Verification items for the finished model (mm, model axes). A direction names the side the tool comes from. Give positions to 0.01 mm unless a question says otherwise; leave off trailing zeros. Write each loop counter-clockwise with the first axis right and the second up, starting at its lowest first coordinate (ties: lowest second). Pieces come first, ordered by that corner, then holes. Notation, with made-up numbers: M -18,53 L -10,53 A23 ccw -10,92 Z; hole C 66.5,-38.5 d9. An arc over 180 degrees is marked long. Write item = value, one per line.
Autodesk Fusion 360 part; units mm, degrees
sketch "Sketch1" plane through (0, 0, 0) normal (1, 0, 0) x (0, 0, -1)
  line L0 (0, 0) -> (0, 45)
  line L1 (0, 0) -> (0, -45)
  line L2 (0, 45) -> (37.5, 45)
  line L3 (0, 45) -> (-37.5, 45)
  line L4 (0, -45) -> (37.5, -45)
  line L5 (0, -45) -> (-37.5, -45)
  arc A0 (-37.5, 45) -> (-37.5, -45) centre (79.119, 0) ccw
  arc A1 (37.5, -45) -> (37.5, 45) centre (-79.119, 0) ccw
  dimension "d1" = 45
  dimension "d2" = 45
  dimension "d3" = 37.5
  dimension "d4" = 37.5
  dimension "d5" = 37.5
  dimension "d6" = 37.5
  dimension "d8" = 125
extrude "Extrude1" add sketch "Sketch1" along normal blind 100
extrude "Extrude2" add 1 faces at (100, -15.2642, -14.2806) along direction (1, 0, 0) blind 35 draft -15
sketch "Sketch2" plane through (135, 0, 0) normal (1, 0, 0) x (0, 0, -1)
  line L0 (-30.8786, -35.6218) -> (30.8786, -35.6218)
  arc A0 (30.8786, -35.6218) -> (30.8786, 35.6218) centre (-79.119, 0) ccw
  line L1 (30.8786, 35.6218) -> (-30.8786, 35.6218)
  arc A1 (-30.8786, 35.6218) -> (-30.8786, -35.6218) centre (79.119, 0) ccw
  circle A2 centre (0, 0) radius 34.5
  dimension "d13" = 69
extrude "Extrude3" add sketch "Sketch2" along normal blind 10 contours A2
sketch "Sketch3" plane through (145, 0, 0) normal (1, 0, 0) x (0, 0, -1)
  circle A0 centre (0, 0) radius 34.5
  circle A1 centre (0, 0) radius 31
  dimension "d16" = 62
extrude "Extrude4" add sketch "Sketch3" along normal blind 30 contours A1
sketch "Sketch4" plane through (175, 0, 0) normal (1, 0, 0) x (0, 0, -1)
  circle A0 centre (0, 0) radius 31
  line L0 (0, 0) -> (27, 0)
  circle A1 centre (27, 0) radius 2.5
  circle A2 centre (27, 0) radius 1.5
  dimension "d19" = 27
  dimension "d20" = 5
  dimension "d21" = -1
extrude "Extrude5" add sketch "Sketch4" along normal blind 1 contours A1
pattern_circular "C-Pattern1" count 12 over 360 about axis through (175, 0, 0) along (1, 0, 0) of "Extrude5"
sketch "Sketch5" plane through (175, 0, 0) normal (1, 0, 0) x (0, 0, -1)
  circle A0 centre (27, 0) radius 2.5
  circle A1 centre (0, 0) radius 31
  circle A2 centre (23.3827, 13.5) radius 2.5
  circle A3 centre (13.5, 23.3827) radius 2.5
  circle A4 centre (0, 27) radius 2.5
  circle A5 centre (-13.5, 23.3827) radius 2.5
  circle A6 centre (-23.3827, 13.5) radius 2.5
  circle A7 centre (-27, 0) radius 2.5
  circle A8 centre (-23.3827, -13.5) radius 2.5
  circle A9 centre (-13.5, -23.3827) radius 2.5
  circle A10 centre (0, -27) radius 2.5
  circle A11 centre (13.5, -23.3827) radius 2.5
  circle A12 centre (23.3827, -13.5) radius 2.5
  line L0 (0, 0) -> (16, 0)
  line L1 (16, 0) -> (16, 17)
  line L2 (16, 0) -> (16, -17)
  line L3 (0, 0) -> (0, -8.0593)
  line L4 (-16, 0) -> (-16, 17)
  line L5 (-16, 0) -> (-16, -17)
  arc A13 (16, 17) -> (-16, 17) centre (0, 1.9003) ccw
  arc A14 (-16, -17) -> (16, -17) centre (0, -1.9003) ccw
  dimension "d26" = 16
  dimension "d27" = 17
  dimension "d28" = 17
  dimension "d29" = 22
extrude "Extrude6" add sketch "Sketch5" along normal blind 100 contours L1 L2 L4 L5 A13 A14
sketch "Sketch6" plane through (275, 0, 0) normal (1, 0, 0) x (0, 0, -1)
  line L0 (-16, 17) -> (-16, -17)
  arc A0 (-16, -17) -> (16, -17) centre (0, -1.9003) ccw
  line L1 (16, -17) -> (16, 17)
  arc A1 (16, 17) -> (-16, 17) centre (0, 1.9003) ccw
  circle A2 centre (0, 0) radius 31
  dimension "d32" = 62
extrude "Extrude7" add sketch "Sketch6" along normal blind 10 contours L0 A0 L1 A1 | A2
1) Cross-section at C-C on x = 232.5. Record the boundary of the cut face in (y, z), plus the area to 3 significant figures.
From the geometry:
outline = M -17,-16 L 17,-16 A22 ccw 17,16 L -17,16 A22 ccw Z
area = 1,390 mm^2
2) Cross-section at A-A on x = 138. Record the boundary of the cut face in (y, z).
From the geometry:
outline = C 0,0 d69
3) Draft check along Y on faces 5 (the cylindrical face through (175.5, -24.5, 0.1)), 6 (the cylindrical face through (175.5, 24.5, -0.1)), 7 (the flat face through (176, 0, 29)), 8 (the flat face through (49, -45, -1)). Enter one of: +Y half, -Y half, draft (parallel to the pull), parting line (faces both ways), or undercut.
From the geometry:
face_5 = undercut
face_6 = undercut
face_7 = draft
face_8 = -Y half
4) Depth check by flat-ended pin: P1, Ø3, axis at x = 128.5, z = -23.5, coming from the +Y side; P2, Ø4, axis at y = 34, z = -27.5, coming from the +X side; P3, Ø10, axis at x = 156.5, y = 30, coming from the +Z side. Enter the tip coordinate at first touch or a pass-through.
From the geometry:
P1 = 37.77
P2 = 135
P3 = 18.33
5) Tool access check on faces 1 (the flat face through (176, -13, 25)), 2 (the cylindrical face through (175.493, -25.823, -14.042)), 3 (the flat face through (176, 25, 13)), 4 (the cylindrical face through (139.93, -10.363, -32.907)). Record the directions out of +Z, -Z, +X, -X, +Y, -Y that give a thin tool (end or side, any length) a straight path to the whole face; none if there is none.
From the geometry:
face_1 = +Z, +Y, -Y
face_2 = none
face_3 = +Z, +Y
face_4 = +X
6) Material ranges on probe 1 along Z at (x, y) = (175.5, 13.5); probe 2 along X at (y, z) = (5, -20.5); probe 3 along X at (y, z) = (-23, -23.5), recorded low to high. Write a range as from..to.
From the geometry:
probe_1 = -25.88..-24.88, -21.88..-20.88, -16..16, 20.88..21.88, 24.88..25.88
probe_2 = 0..175, 275..285
probe_3 = 0..145
7) Cross-section at B-B on x = 83. Record the boundary of the cut face in (y, z).
From the geometry:
outline = M -45,-37.5 A125 ccw 45,-37.5 L 45,37.5 A125 ccw -45,37.5 Z
